from build123d import *

# Parameters (mm, degrees)
BOSS_EXTRUDE1_DEPTH               = 60.325
BOSS_EXTRUDE2_START               = -64.325
SKETCH4_R                         = 10
BOSS_EXTRUDE2_DEPTH               = 68.325
SKETCH5_R                         = 5.159375
CUT_EXTRUDE1_DEPTH                = 69.325
SKETCH6_W                         = 75.649114878
SKETCH6_H                         = 60.325
BOSS_EXTRUDE3_DEPTH               = 1.8288
BOSS_EXTRUDE4_REACH               = 190.905
BOSS_EXTRUDE4_OFFSET_FROM_SURFACE = 49
SKETCH8_R                         = 30
SKETCH9_R                         = 15.5
CUT_EXTRUDE2_DEPTH                = 190.266787166
CUT_EXTRUDE3_DEPTH                = 49
SKETCH11_W                        = 50.325
SKETCH11_H                        = 86.143116626
CUT_EXTRUDE4_DEPTH                = 109.525496818
SKETCH15_R                        = 3.175
CUT_EXTRUDE5_DEPTH                = 190.266787166
FILLET1_R                         = 3.81


with BuildPart() as part:
    # Sketch2 → Boss-Extrude1 (new body)
    with BuildSketch(Plane.XY):
        with BuildLine():
            Line((12.765629792, 129.146573189), (-1.754589441, 128.968962917))
            Line((-1.754589441, 128.968962917), (-1.754589441, 83.82382539))
            Line((-1.754589441, 83.82382539), (20.592124083, 68.316599476))
            Line((20.592124083, 68.316599476), (20.592124083, 36.846052768))
            Line((20.592124083, 36.846052768), (-2.252403515, 21.475974179))
            Line((-2.252403515, 21.475974179), (-2.252403515, 12.414958495))
            Line((-2.252403515, 12.414958495), (-2.252403515, -8.161795964))
            Line((-2.252403515, -8.161795964), (75.649114878, -8.161795964))
            Line((75.649114878, -8.161795964), (73.96041286, 129.895103354))
            Line((73.96041286, 129.895103354), (24.530310461, 129.290477913))
            Line((24.530310461, 129.290477913), (24.530310461, 114.148644142))
            ThreePointArc((24.530310461, 114.148644142), (18.82597029, 108.263437866), (12.765629792, 113.781356201))
            ThreePointArc((12.765629792, 113.781356201), (12.754163231, 114.148644142), (12.765629792, 114.515932083))
            Line((12.765629792, 114.515932083), (12.765629792, 129.146573189))
        make_face()
    extrude(amount=BOSS_EXTRUDE1_DEPTH)

    # Sketch4 → Boss-Extrude2 (add)
    with BuildSketch(Plane.XY.offset(60.325).offset(BOSS_EXTRUDE2_START)):
        Circle(SKETCH4_R)
    extrude(amount=BOSS_EXTRUDE2_DEPTH)

    # Sketch5 → Cut-Extrude1 (cut, through all)
    with BuildSketch(Plane.XY.offset(64.325)):
        Circle(SKETCH5_R)
    extrude(amount=-CUT_EXTRUDE1_DEPTH, mode=Mode.SUBTRACT)

    # Sketch6 → Boss-Extrude3 (add)
    with BuildSketch(Plane.XZ.offset(8.161795964)):
        with Locations((37.824557439, 30.1625)):
            Rectangle(SKETCH6_W, SKETCH6_H)
    extrude(amount=BOSS_EXTRUDE3_DEPTH)

    # Boss-Extrude4: up to this face of the body (flat: up to its plane, moved by the offset)
    boss_extrude4_end = Plane(part.part.faces().sort_by_distance((38.041347827, -9.990595964, 30.1625))[0]).offset(BOSS_EXTRUDE4_OFFSET_FROM_SURFACE)
    # Sketch8 → Boss-Extrude4 (add, up to the picked face)
    with BuildSketch(Plane(origin=(-1.577565522, 128.97112826, 0), x_dir=(0.999925198, 0.012231013, 0), z_dir=(-0.012231013, 0.999925198, 0)), mode=Mode.PRIVATE) as boss_extrude4_sk1:
        with Locations((75.543629169, -30.1625)):
            Circle(SKETCH8_R)
    boss_extrude4_tool1 = split(extrude(boss_extrude4_sk1.sketch, amount=-BOSS_EXTRUDE4_REACH, mode=Mode.PRIVATE), bisect_by=boss_extrude4_end, keep=Keep.BOTH, mode=Mode.PRIVATE)
    add(boss_extrude4_tool1.solids().sort_by_distance((73.960413, 129.895103, 30.1625))[0])

    # Sketch9 → Cut-Extrude2 (cut, through all)
    with BuildSketch(Plane(origin=(-1.577565522, 128.97112826, 0), x_dir=(0.999925198, 0.012231013, 0), z_dir=(-0.012231013, 0.999925198, 0))):
        with Locations((75.543629169, -30.1625)):
            Circle(SKETCH9_R)
    extrude(amount=-CUT_EXTRUDE2_DEPTH, mode=Mode.SUBTRACT)

    # Sketch10 → Cut-Extrude3 (cut)
    with BuildSketch(Plane.ZY.offset(-125.245410559)):
        Polygon((60.325, 109.914722857), (60.1625, -38.990595964), (-4.123053696, -38.990595964), (-4.123053696, 109.914722857), align=None)
    extrude(amount=CUT_EXTRUDE3_DEPTH, mode=Mode.SUBTRACT)

    # Sketch11 → Cut-Extrude4 (cut, through all)
    with BuildSketch(Plane.ZY.offset(2.252403515)):
        with Locations((30.1625, 53.897404604)):
            Rectangle(SKETCH11_W, SKETCH11_H)
    extrude(amount=-CUT_EXTRUDE4_DEPTH, mode=Mode.SUBTRACT)

    # Sketch15 → Cut-Extrude5 (cut, through all)
    with BuildSketch(Plane(origin=(-1.577565522, 128.97112826, 0), x_dir=(0.999925198, 0.012231013, 0), z_dir=(-0.012231013, 0.999925198, 0))):
        with Locations((20.227048665, -30.1625)):
            Circle(SKETCH15_R)
    extrude(amount=-CUT_EXTRUDE5_DEPTH, mode=Mode.SUBTRACT)

    # Fillet1
    fillet1_edges = [part.edges().sort_by_distance(p)[0] for p in [
        (-2.252403515, 21.475974179, 2.5),
        (20.592124083, 36.846052768, 2.5),
        (20.592124083, 68.316599476, 2.5),
        (-1.754589441, 83.82382539, 2.5),
        (-2.252403515, 21.475974179, 57.825),
        (20.592124083, 36.846052768, 57.825),
        (20.592124083, 68.316599476, 57.825),
        (-1.754589441, 83.82382539, 57.825),
    ]]
    fillet(fillet1_edges, radius=FILLET1_R)


solid = part.part
Read the model definition and answer for the solid it produces. Units are mm, in the model's axes. A direction names the side the tool comes from. Give positions to 0.01 mm unless a question says otherwise; leave off trailing zeros. Loops run counter-clockwise (first coordinate to the right, second up) from the corner with the lowest first, then second, coordinate; pieces in that order, holes last. Notation, with made-up numbers: M 66,30.25 L 94,30.25 A16 ccw 94,54.25 Z; hole C 88,-10.75 d4. An arc over 180 degrees is marked long. Write each question's results on one line, items separated by ' | '.
1. Section B-B on z = 10 is taken. Give the vertices of the cut face in (x, y), plus the area to 3 significant figures.
Values:
outline: M -2.25,9.74 A10 ccw 0.43,-9.99 L 53.46,-9.99 L 54.05,-58.99 L 98.49,-58.99 L 98.24,-38.99 L 76.25,-38.99 L 76.25,10.83 L -2.25,10.83 Z; M -1.75,96.97 L 76.25,96.97 L 76.25,109.91 L 96.42,109.91 L 96.17,130.17 L 24.53,129.29 L 24.53,114.15 A5.89 cw long 12.77,114.52 L 12.77,129.15 L -1.75,128.97 Z; hole C 0,0 d10.32 | area: 5,910 mm^2
2. The mould has two halves that part along Y. Classify faces 5 (the face through (45, 53, 5)), 6 (the face through (29, -9.991, 31)), 7 (the face through (9.29, 76.16, 2.46)), 8 (the face through (-2.252, 10, 30)): pulls with the +Y half, pulls with the -Y half, needs draft (parallel to the pull), parting line crosses it, or undercut.
Values:
face 5: undercut | face 6: pulls with the -Y half | face 7: undercut | face 8: needs draft
3. Section D-D on z = 53 is taken. Give the vertices of the cut face in (x, y).
Values:
outline: M -2.25,9.74 A10 ccw 0.43,-9.99 L 56.22,-9.99 L 56.82,-58.99 L 95.73,-58.99 L 95.48,-38.99 L 76.25,-38.99 L 76.25,10.83 L -2.25,10.83 Z; M -1.75,96.97 L 76.25,96.97 L 76.25,109.91 L 93.66,109.91 L 93.41,130.13 L 24.53,129.29 L 24.53,114.15 A5.89 cw long 12.77,114.52 L 12.77,129.15 L -1.75,128.97 Z; hole C 0,0 d10.32
4. Section A-A on z = 20 is taken. Give the vertices of the cut face in (x, y).
Values:
outline: M -2.25,9.74 A10 ccw 0.43,-9.99 L 47.44,-9.99 L 48.04,-58.99 L 64.57,-58.99 L 63.71,10.83 L -2.25,10.83 Z; M -1.75,96.97 L 62.66,96.97 L 62.26,129.75 L 24.53,129.29 L 24.53,114.15 A5.89 cw long 12.77,114.52 L 12.77,129.15 L -1.75,128.97 Z; M 85.66,130.04 L 85.91,109.91 L 102.43,109.91 L 102.18,130.24 Z; M 87.73,-38.99 L 87.98,-58.99 L 104.5,-58.99 L 104.25,-38.99 Z; hole C 0,0 d10.32
5. Section C-C on y = 0 is taken. State how many separate pieces and enclosed holes the cut face has, plus the area to 3 significant figures.
Values:
separate pieces: 2 | enclosed holes: 1 | area: 4,230 mm^2
6. Given pin 1 (14 mm diameter, centred on x = 84, z = 22.5, fed in from -Y); pin 2 (8 mm diameter, centred on x = 50, y = 54.5, fed in from +Z) (3 decimals); pin 3 (7.5 mm diameter, centred on y = 21, z = 7.5, fed in from +X); pin 4 (10 mm diameter, centred on x = 43, y = 108.5, fed in from -Z), each flat-ended and moving along its own axis, determine where each tip first touches the part or whether it passes through.
Values:
pin 1: stops at y = -58.99 | pin 2: stops at z = 60.325 | pin 3: stops at x = 76.25 | pin 4: stops at z = 0
7. Straight lines are drawn through the part: line 1 (Y direction, x = 0, z = 29); line 2 (Y direction, x = -1.5, z = 21.5); line 3 (Z direction, x = 72, y = 62.5) (3 decimals). For each, find the intervals that lie inside material, in ascending order. Write a range as [from, to].
Values:
line 1: y = [-10, -5.16], [5.16, 10.83], [96.97, 128.99] | line 2: y = [-9.89, -4.94], [4.94, 10.83], [96.97, 128.97] | line 3: z = [0, 5], [55.325, 60.325]
8. A tool of negligible diameter and unlimited length cuts with its end or side. For faces 1 (the face through (58.63, 117.12, 29.48)), 2 (the face through (95, -38.991, 31)), 3 (the face through (36, 10.826, 30)), 4 (the face through (24.53, 122, 30)), from which of +Z, -Z, +X, -X, +Y, -Y can it reach the whole face along a straight path? Write none if from no direction.
Values:
face 1: none | face 2: +Z, -Z, +X | face 3: +X, -X | face 4: +Z, -Z, +Y
